Could you check a few things on this model? Use its own coordinates, in mm. Round coordinates to 2 decimals unless told otherwise and drop trailing zeros. Order: outer loops, then holes, each group sorted by start corner. A loop starts at its lowest first (then second) coordinate and runs counter-clockwise, first axis right, second up.
```python
from build123d import *

# Parameters (mm, degrees)
SKETCH1_R          = 3.1
EXTRUDE1_DEPTH     = 0.7
SKETCH2_R          = 1.7
CUT_EXTRUDE1_DEPTH = 5.439594576
SKETCH3_W          = 1.509479926
SKETCH3_H          = 0.191482381
CUT_EXTRUDE3_DEPTH = 5.439594576


with BuildPart() as part:
    # Sketch1 → Extrude1 (new body)
    with BuildSketch(Plane(origin=(0, 0, 0), x_dir=(1, 0, 0), z_dir=(0, 1, 0))):
        with Locations(Location((0, 0, 0), (0, 0, 270))):
            Circle(SKETCH1_R)
    extrude(amount=EXTRUDE1_DEPTH)

    # Sketch2 → Cut-Extrude1 (cut, through all)
    with BuildSketch(Plane(origin=(0, 0.7, 0), x_dir=(1, 0, 0), z_dir=(0, 1, 0))):
        with Locations(Location((0, 0, 0), (0, 0, 270))):
            Circle(SKETCH2_R)
    extrude(amount=-CUT_EXTRUDE1_DEPTH, mode=Mode.SUBTRACT)

    # Sketch3 → Cut-Extrude3 (cut, through all)
    with BuildSketch(Plane(origin=(0, 0.7, 0), x_dir=(1, 0, 0), z_dir=(0, 1, 0))):
        with Locations((2.450921504, 0.018136723)):
            Rectangle(SKETCH3_W, SKETCH3_H)
    extrude(amount=-CUT_EXTRUDE3_DEPTH, mode=Mode.SUBTRACT)


solid = part.part
```
Q1. Imagine slicing it at B-B, the plane z = 0.5. Please give me the cut outline in (x, y).
Q2. We'd pull the mould along X, two halves only. Please class faces 1 (the flat face through (-1.33, 0, 1.33)), 2 (the cylindrical face through (-1.7, 0.35, -0.06)): released by +X, released by -X, zero draft, split by the parting line, or undercut.
Q3. Imagine slicing it at D-D, the plane z = 2.75. Please give me the cut outline in (x, y).
Q4. Imagine slicing it at C-C, the plane y = 0.35. Please give me the cut outline in (x, z).
Q5. I need wall thicknesses on L1, parallel to Z at x = 0, y = 0.3; L2, parallel to X at y = 0.2, z = 0; L3, parallel to X at y = 0.35, z = -0.5. Which ranges of each line are inside material? Lowest first, please.
Q6. Imagine slicing it at A-A, the plane x = 1.5. Please give me the cut outline in (y, z).
Filled in:
1. outline: (-3.06, 0) - (-1.62, 0) - (-1.62, 0.7) - (-3.06, 0.7) - close; (1.62, 0) - (3.06, 0) - (3.06, 0.7) - (1.62, 0.7) - close
2. face 1: zero draft
2. face 2: undercut
3. outline: (-1.43, 0) - (1.43, 0) - (1.43, 0.7) - (-1.43, 0.7) - close
4. outline: (1.7, -0.11) arc R1.7 cw (long way) to (1.7, 0.08) - (3.1, 0.08) arc R3.1 ccw (long way) to (3.1, -0.11) - close
5. L1: z = -3.1 to -1.7, 1.7 to 3.1
5. L2: x = -3.1 to -1.7
5. L3: x = -3.06 to -1.62, 1.62 to 3.06
6. outline: (0, -2.71) - (0.7, -2.71) - (0.7, -0.8) - (0, -0.8) - close; (0, 0.8) - (0.7, 0.8) - (0.7, 2.71) - (0, 2.71) - close
